The listing builds one solid part. Answer for the finished solid, in the listing's coordinates (mm). Give positions to 0.01 mm unless a question says otherwise; leave off trailing zeros. Order: outer loops, then holes, each group sorted by start corner. A loop starts at its lowest first (then second) coordinate and runs counter-clockwise, first axis right, second up.
```python
from build123d import *

# Parameters (mm, degrees)
EXTRUDE_START       = 10.8
EXTRUDE_1_DEPTH     = 19.9
SKETCH_2_R          = 0.75
CUT_EXTRUDE_1_DEPTH = 20.9


with BuildPart() as part:
    # Эскиз1 → Бобышка-Вытянуть1 (new body)
    with BuildSketch(Plane(origin=(0, 0, 0), x_dir=(1, 0, 0), z_dir=(0, 1, 0)).offset(EXTRUDE_START)):
        Polygon((2.886751346, 0), (1.443375673, 2.5), (-1.443375673, 2.5), (-2.886751346, 0), (-1.443375673, -2.5), (1.443375673, -2.5), align=None)
    extrude(amount=EXTRUDE_1_DEPTH)

    # Эскиз2 → Вырез-Вытянуть1 (cut, through all)
    with BuildSketch(Plane(origin=(0, 30.7, 0), x_dir=(1, 0, 0), z_dir=(0, 1, 0))):
        Circle(SKETCH_2_R)
    extrude(amount=-CUT_EXTRUDE_1_DEPTH, mode=Mode.SUBTRACT)


solid = part.part
```
1) Find section D-D (x = 2.2). Write down the section's boundary in (y, z).
Geometry says:
outline: (10.8, -1.19) - (30.7, -1.19) - (30.7, 1.19) - (10.8, 1.19) - close
2) Given P1, Ø1.7, axis at x = 0, z = 0, coming from the +Y side, flat-ended and moving along its own axis, determine where the tip first touches the part or whether it passes through.
Geometry says:
P1: stops at y = 30.7
3) Straight lines are drawn through the part: probe 1 along Z at (x, y) = (0, 20); probe 2 along X at (y, z) = (23.5, -0.1); probe 3 along X at (y, z) = (16.25, 1.6). For each, find the intervals that lie inside material, in ascending order.
Geometry says:
probe 1: z = -2.5 to -0.75, 0.75 to 2.5
probe 2: x = -2.83 to -0.74, 0.74 to 2.83
probe 3: x = -1.96 to 1.96
4) Find section A-A (x = 0). Write down the section's boundary in (y, z).
Geometry says:
outline: (10.8, -2.5) - (30.7, -2.5) - (30.7, -0.75) - (10.8, -0.75) - close; (10.8, 0.75) - (30.7, 0.75) - (30.7, 2.5) - (10.8, 2.5) - close
5) Find section B-B (y = 29.75). Write down the section's boundary in (x, z), then the cut area to 3 significant figures.
Geometry says:
outline: (-2.89, 0) - (-1.44, -2.5) - (1.44, -2.5) - (2.89, 0) - (1.44, 2.5) - (-1.44, 2.5) - close; hole circle Ø1.5 at (0, 0)
area: 19.9 mm2
6) Find section C-C (z = 1.15). Write down the section's boundary in (x, y).
Geometry says:
outline: (-2.22, 10.8) - (2.22, 10.8) - (2.22, 30.7) - (-2.22, 30.7) - close
